Answer from the drawing. Dimensions are ordinates in mm from the lowest x, y and z of the part. Coordinates: 2 decimals unless noted, no trailing zeros. Order: outer loops, then holes, each group sorted by start corner. A loop starts at its lowest first (then second) coordinate and runs counter-clockwise, first axis right, second up. Notation, with made-up numbers: (-28, 54.25) - (-17, 54.25) arc R22 cw to (-17, 82.25) - close; hole circle Ø4 at (11, -12). An arc over 180 degrees is marked (long way). One line per item, written item: value. Start each with the question number.
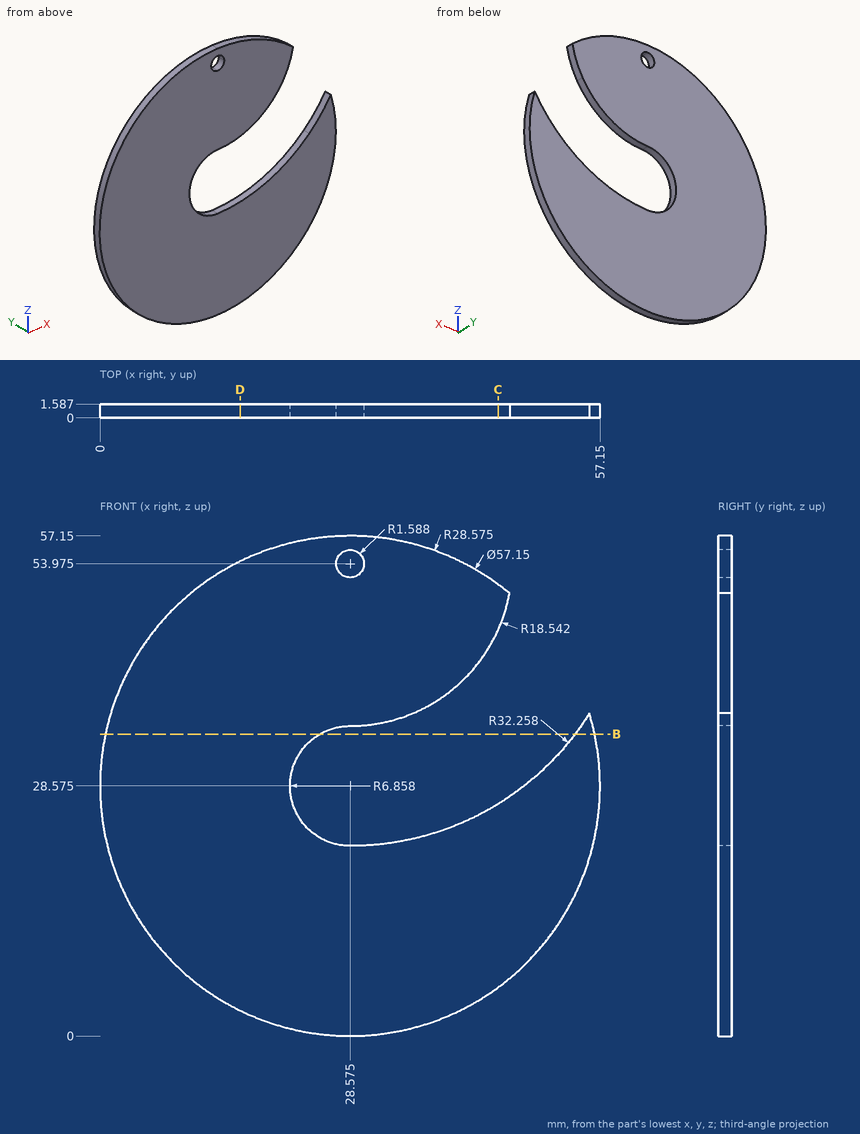
(1) The part is cut by section B-B on z = 34.5. Determine the outline of the cut face in (x, y).
(2) Consider probe 1 along X at (y, z) = (0.15, 34) (1 decimal); probe 2 along Z at (x, y) = (26, 0.5) (1 decimal); probe 3 along X at (y, z) = (0.6, 21.5). Determine where each line is inside the solid, lowest interval first.
(3) The part is cut by section D-D on x = 16. Determine the outline of the cut face in (y, z) (1 decimal).
(4) The part is cut by section C-C on x = 45.5. Determine the outline of the cut face in (y, z).
Completed:
1. outline: (0.62, 0) - (25.12, 0) - (25.12, 1.59) - (0.62, 1.59) - close; (54.29, 0) - (56.53, 0) - (56.53, 1.59) - (54.29, 1.59) - close
2. probe 1: x = 0.5 to 24.4, 53.9 to 56.6
2. probe 2: z = 0.1 to 22.2, 34.9 to 57
2. probe 3: x = 0.89 to 56.26
3. outline: (0, 2.9) - (1.6, 2.9) - (1.6, 54.2) - (0, 54.2) - close
4. outline: (0, 5.55) - (1.59, 5.55) - (1.59, 26.51) - (0, 26.51) - close; (0, 46.4) - (1.59, 46.4) - (1.59, 51.6) - (0, 51.6) - close
